Could you check a few things on this model? Use its own coordinates, in mm. A direction names the side the tool comes from. Give positions to 0.01 mm unless a question says otherwise; leave off trailing zeros. Order: outer loops, then holes, each group sorted by start corner. A loop starts at its lowest first (then second) coordinate and runs counter-clockwise, first axis right, second up. Notation, with made-up numbers: M 2,35 L 21,35 A17 cw 21,60 Z; hole C -15.5,56 d6. An arc over 180 degrees is marked long. Return JSON: item names as keys, results as strings. Group by question number.
```python
from build123d import *

# Parameters (mm, degrees)
SKETCH1_W           = 150
SKETCH1_H           = 160
BOSS_EXTRUDE1_DEPTH = 16
SKETCH4_R           = 4
SKETCH4_W           = 22.5
SKETCH4_H           = 22.5
CUT_EXTRUDE1_DEPTH  = 17


with BuildPart() as part:
    # Sketch1 → Boss-Extrude1 (new body)
    with BuildSketch(Plane.XY):
        Rectangle(SKETCH1_W, SKETCH1_H)
    extrude(amount=BOSS_EXTRUDE1_DEPTH)

    # Sketch4 → Cut-Extrude1 (cut, through all)
    with BuildSketch(Plane.XY.offset(16)):
        with Locations((-62, 65)):
            Circle(SKETCH4_R)
        with Locations((62, 65)):
            Circle(SKETCH4_R)
        with Locations((62, -65)):
            Circle(SKETCH4_R)
        with Locations((-62, -65)):
            Circle(SKETCH4_R)
        with Locations((-38.75, 38.75)):
            Rectangle(SKETCH4_W, SKETCH4_H)
        with Locations((38.75, 38.75)):
            Rectangle(SKETCH4_W, SKETCH4_H)
        with Locations((-38.75, -48.75)):
            Rectangle(SKETCH4_W, SKETCH4_H)
        with Locations((38.75, -48.75)):
            Rectangle(SKETCH4_W, SKETCH4_H)
        with Locations((-38.75, -5)):
            Rectangle(SKETCH4_W, SKETCH4_H)
        with Locations((38.75, -5)):
            Rectangle(SKETCH4_W, SKETCH4_H)
    extrude(amount=-CUT_EXTRUDE1_DEPTH, mode=Mode.SUBTRACT)


solid = part.part
```
1. Imagine slicing it at B-B, the plane y = -40.5. Please give me the cut outline in (x, z), plus the area to 3 significant figures.
2. Which directions (+Z, -Z, +X, -X, +Y, -Y) give clear straight access to the entire face, cutting with the end or side of a thin tool? Please do faces 3 (the flat face through (-75, -1, 8)), 4 (the flat face through (-39, 27.5, 8)).
3. Imagine slicing it at A-A, the plane x = -62. Please give me the cut outline in (y, z).
4. If we mould it in two halves opening along Y, with no side actions, what happens to faces 1 (the flat face through (27.5, 39, 8)), 2 (the flat face through (-1, 1, 0))? For each: pulls with the +Y half, pulls with the -Y half, needs draft (parallel to the pull), parting line crosses it, or undercut.
5. Imagine slicing it at C-C, the plane z = 7.75. Count the separate pieces of the cut face and the enclosed holes in it, plus the area to 3 significant figures.
6. I need wall thicknesses on L1, parallel to Y at x = 47, z = 5.75; L2, parallel to Y at x = 62, z = 7.5; L3, parallel to X at y = -54, z = 10.5. Which ranges of each line are inside material? Lowest first, please. Write a range as from..to.
Values:
{
 "1": {"outline": "M -75,0 L -50,0 L -50,16 L -75,16 Z; M -27.5,0 L 27.5,0 L 27.5,16 L -27.5,16 Z; M 50,0 L 75,0 L 75,16 L 50,16 Z", "area": "1,680 mm²"},
 "2": {"face 3": "+Z, -Z, -X, +Y, -Y", "face 4": "+Z, -Z"},
 "3": {"outline": "M -80,0 L -69,0 L -69,16 L -80,16 Z; M -61,0 L 61,0 L 61,16 L -61,16 Z; M 69,0 L 80,0 L 80,16 L 69,16 Z"},
 "4": {"face 1": "undercut", "face 2": "needs draft"},
 "5": {"separate pieces": "1", "enclosed holes": "10", "area": "20,800 mm²"},
 "6": {"L1": "y = -80..-60, -37.5..-16.25, 6.25..27.5, 50..80", "L2": "y = -80..-69, -61..61, 69..80", "L3": "x = -75..-50, -27.5..27.5, 50..75"}
}
